Autodesk Inventor part; units mm, degrees
ref_plane "YZ Plane" through (0, 0, 0) normal (1, 0, 0) x (0, 1, 0)
ref_plane "XZ Plane" through (0, 0, 0) normal (0, 1, 0) x (-1, 0, 0)
ref_plane "XY Plane" through (0, 0, 0) normal (0, 0, 1) x (1, 0, 0)
sketch "Sketch1" plane through (0, 0, 0) normal (0, 1, 0) x (-1, 0, 0)
  line L0 (0, 0) -> (-25, 0)
  line L1 (-25, 0) -> (-25, -10)
  line L2 (-25, -10) -> (-15, -10)
  line L3 (-15, -10) -> (-15, -45)
  line L4 (-15, -45) -> (0, -45)
  line L5 (0, 0) -> (0, -45)
  dimension "d3" = 25
  dimension "d4" = 10
  dimension "d5" = 10
  dimension "d6" = 35
  dimension "d7" = 15
revolve "Revolution1" add sketch "Sketch1" angle 360 about axis through (0, 0, 0) along (0, 0, -1)
sketch "Sketch2" plane through (0, 0, 0) normal (0, 0, 1) x (1, 0, 0)
  line L0 (0, 0) -> (30.242, 0) construction
  line L1 (0, 0.5707) -> (22.435, 0.5707) construction
  circle A0 centre (9.7519, 17.4614) radius 2.25
  circle A1 centre (19.998, 0.2854) radius 2.25
  circle A2 centre (10.2461, -17.1761) radius 2.25
  circle A3 centre (-9.7519, -17.4614) radius 2.25
  circle A4 centre (-19.998, -0.2854) radius 2.25
  circle A5 centre (-10.2461, 17.1761) radius 2.25
  dimension "d12" = 4.5
  dimension "d15" = 360
extrude "Extrusion1" cut sketch "Sketch2" against normal through all
sketch "Sketch3" plane through (0, 0, 0) normal (0, 0, 1) x (1, 0, 0)
  circle A0 centre (0, 0) radius 5.5
  dimension "d19" = 11
extrude "Extrusion2" cut sketch "Sketch3" against normal through all
thread "Thread1"
properties part number "nut"
Can you work these out from the model? Positions are in its coordinate system, mm. A direction names the side the tool comes from. Coordinates: 2 decimals unless noted, no trailing zeros. Write each loop counter-clockwise with the first axis right and the second up, starting at its lowest first coordinate (ties: lowest second). Pieces come first, ordered by that corner, then holes. Notation, with made-up numbers: M 49,-30.5 L 78,-30.5 A12 ccw 78,-7.5 Z; hole C 68,62.5 d3. An arc over 180 degrees is marked long. Write item = value, one per line. Start each with the question number.
Q1. If we section it at B-B, the plane z = -21: Write out the boundary of the cut face in (x, y), then the cut area to 3 significant figures.
Q2. I'm going to push flat-ended pins straight in: pin 1 (2 mm diameter, centred on y = 2.5, z = -22.5, fed in from +X); pin 2 (8 mm diameter, centred on x = -13.5, z = -28.5, fed in from +Y); pin 3 (8 mm diameter, centred on y = 16.5, z = -36.5, fed in from +X). Where does each tip first touch, or does it pass through?
Q3. On a 3-axis mill with a long thin cutter (end or side, diameter ignored), from which of +Z, -Z, +X, -X, +Y, -Y can I reach the whole of each face in a straight line? I mean faces 1 (the face through (11, 11, -10)), 2 (the face through (-22.246, -0.186, -4.93)). Say none if no direction works.
Q4. If we section it at C-C, the plane x = 10: Write out the boundary of the cut face in (y, z).
Q5. If we section it at D-D, the plane y = 7: Write out the boundary of the cut face in (x, z), then the cut area to 3 significant figures.
Q6. If I drill on L1, parallel to Y at x = -10.5, z = -6; L2, parallel to Y at x = 18.5, z = -2.5; L3, parallel to Z at x = -16, y = -2.5, over which ranges is the centre line in solid material (lowest first)? Write a range as [from, to].
Q7. Thinking about a two-plate mould opening in Y: for faces 3 (the face through (-6, 0, 0)), 4 (the face through (11.46, -15.28, -4.93)), 5 (the face through (18.34, 1.806, -4.93)), 6 (the face through (23.846, -7.509, -5.07)), which applies, released by +Y, released by -Y, zero draft, split by the parting line, or undercut?
Q8. If we section it at A-A, the plane x = 0: Write out the boundary of the cut face in (y, z).
Check sheet entries:
q1.outline = C 0,0 d30; hole C 0,0 d11
q1.area = 612 mm²
q2.pin_1 = 14.92
q2.pin_2 = 11.61
q2.pin_3 = 8.29
q3.face_1 = -Z
q3.face_2 = +Z, -Z
q4.outline = M -22.91,-10 L -19.41,-10 L -19.41,0 L -22.91,0 Z; M -14.94,-10 L -11.18,-10 L -11.18,-45 L 11.18,-45 L 11.18,-10 L 15.23,-10 L 15.23,0 L -14.94,0 Z; M 19.7,-10 L 22.91,-10 L 22.91,0 L 19.7,0 Z
q5.outline = M -24,-10 L -13.27,-10 L -13.27,-45 L 13.27,-45 L 13.27,-10 L 24,-10 L 24,0 L -24,0 Z
q5.area = 1,410 mm²
q6.L1 = [-22.69, -19.58], [-15.34, 14.94], [19.41, 22.69]
q6.L2 = [-16.82, -1.39], [1.96, 16.82]
q6.L3 = [-10, 0]
q7.face_3 = zero draft
q7.face_4 = undercut
q7.face_5 = undercut
q7.face_6 = split by the parting line
q8.outline = M -25,-10 L -15,-10 L -15,-45 L -5.5,-45 L -5.5,0 L -25,0 Z; M 5.5,-45 L 15,-45 L 15,-10 L 25,-10 L 25,0 L 5.5,0 Z
